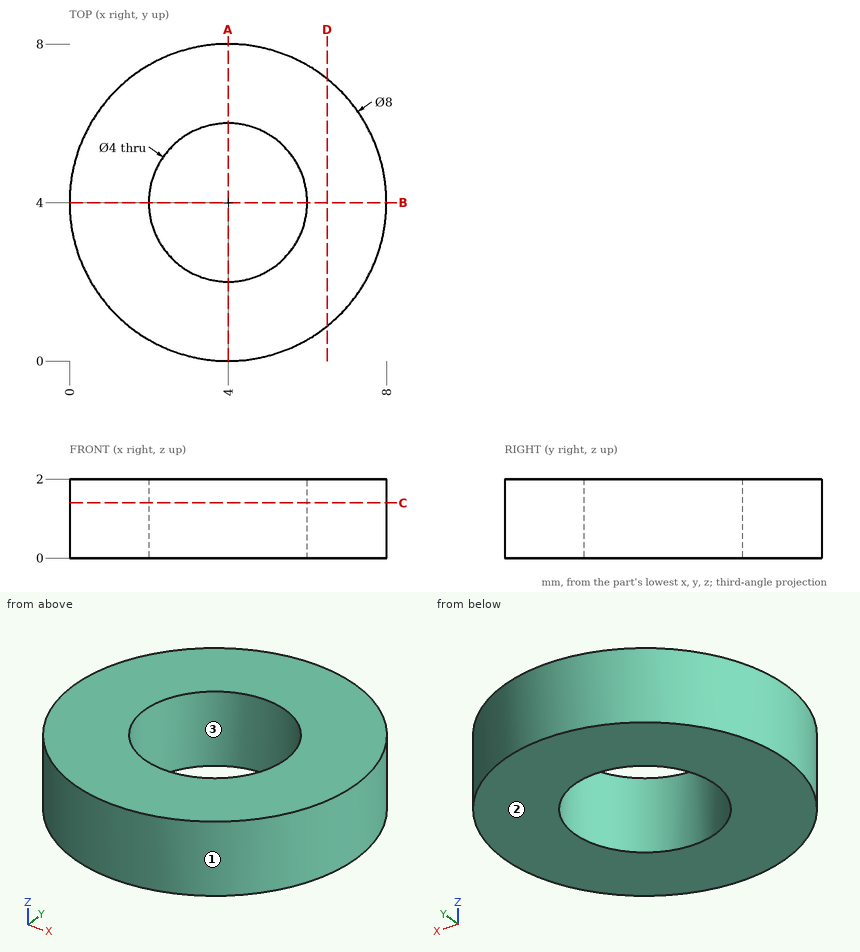
Could you check a few things on this drawing? It's one solid part, dimensions in mm from its lowest x, y, z. Give positions to 0.01 mm unless a question says otherwise; leave off trailing zeros. Loops run counter-clockwise (first coordinate to the right, second up) from the corner with the lowest first, then second, coordinate; pieces in that order, holes last. Notation, with made-up numbers: M -4.75,26.5 L 5.25,26.5 A17 ccw 5.25,56.5 Z; hole C 70,17.5 d8. An arc over 180 degrees is marked long. One line per question, with ' | ' between items. Start each with the question number.
Q1. If we section it at A-A (x = 4): Please give me the cut outline in (y, z).
Q2. If we section it at C-C (z = 1.4): Please give me the cut outline in (x, y).
Q3. If we mould it in two halves opening along Y, with no side actions, what happens to the marked faces 1, 2 and 3? For each: +Y half, -Y half, draft (parallel to the pull), parting line (faces both ways), or undercut.
Q4. If we section it at D-D (x = 6.5): Please give me the cut outline in (y, z), plus the area to 3 significant figures.
Q5. If I drill on line 1 (Y direction, x = 4, z = 0.4); line 2 (X direction, y = 2.25, z = 1.8); line 3 (Y direction, x = 5.5, z = 1.2), over which ranges is the centre line in solid material (lowest first)? Write a range as from..to.
Computed:
1) outline: M 0,0 L 2,0 L 2,2 L 0,2 Z; M 6,0 L 8,0 L 8,2 L 6,2 Z
2) outline: C 4,4 d8; hole C 4,4 d4
3) face 1: parting line | face 2: draft | face 3: undercut
4) outline: M 0.88,0 L 7.12,0 L 7.12,2 L 0.88,2 Z | area: 12.5 mm²
5) line 1: y = 0..2, 6..8 | line 2: x = 0.4..3.03, 4.97..7.6 | line 3: y = 0.29..2.68, 5.32..7.71
